from build123d import *

# Parameters (mm, degrees)
SKETCH035_W      = 36
SKETCH035_H      = 4
EXTRUDE033_DEPTH = 2
SKETCH029_W      = 51.25
SKETCH029_H      = 5
EXTRUDE027_DEPTH = 2
SKETCH017_W      = 8.15
SKETCH017_H      = 2.65
EXTRUDE013_DEPTH = 2
SKETCH010_W      = 14.7
SKETCH010_H      = 2.65
SKETCH010_W_2    = 23.15
SKETCH010_H_2    = 3.15
EXTRUDE006_DEPTH = 2
SKETCH_R         = 1.65
EXTRUDE026_DEPTH = 5
SKETCH009_W      = 51.25
SKETCH009_H      = 53
SKETCH009_W_2    = 47.25
SKETCH009_H_2    = 49
EXTRUDE004_DEPTH = 10.25
SKETCH008_W      = 51.25
SKETCH008_H      = 53
EXTRUDE003_DEPTH = 2
SKETCH028_W      = 5
SKETCH028_H      = 5
EXTRUDE025_DEPTH = 5
SKETCH012_R      = 3
EXTRUDE008_DEPTH = 5


with BuildPart() as topcut002:
    # Sketch035 → Extrude033 (new body)
    with BuildSketch(Plane.YZ.offset(49.25)):
        with Locations((26, 7)):
            Rectangle(SKETCH035_W, SKETCH035_H)
    extrude(amount=EXTRUDE033_DEPTH)


with BuildPart() as top006:
    # Sketch029 → Extrude027 (new body)
    with BuildSketch(Plane.XY.offset(12.25)):
        with Locations((25.625, 2.5)):
            Rectangle(SKETCH029_W, SKETCH029_H)
        with Locations((25.625, 50.5)):
            Rectangle(SKETCH029_W, SKETCH029_H)
    extrude(amount=EXTRUDE027_DEPTH)


with BuildPart() as topcut001:
    # Sketch017 → Extrude013 (new body)
    with BuildSketch(Plane.XZ):
        with Locations((37.575, 6.475)):
            Rectangle(SKETCH017_W, SKETCH017_H)
    extrude(amount=-EXTRUDE013_DEPTH)


with BuildPart() as topcuts:
    # Sketch010 → Extrude006 (new body)
    with BuildSketch(Plane.XZ):
        with Locations((10.5, 3.325)):
            Rectangle(SKETCH010_W, SKETCH010_H)
        with Locations((37.575, 3.575)):
            Rectangle(SKETCH010_W_2, SKETCH010_H_2)
    extrude(amount=-EXTRUDE006_DEPTH)


with BuildPart() as topcuts001:
    # Sketch → Extrude026 (new body)
    with BuildSketch(Plane.XY.offset(10.25)):
        with Locations((22.75, 26.5)):
            Circle(SKETCH_R)
    extrude(amount=-EXTRUDE026_DEPTH)

    # Fusion007: union topCut001, topCuts
    add(topcut001.part)
    add(topcuts.part)


with BuildPart() as top:
    # Sketch009 → Extrude004 (new body)
    with BuildSketch(Plane.XY):
        with Locations((25.625, 26.5)):
            Rectangle(SKETCH009_W, SKETCH009_H)
        with Locations((25.625, 26.5)):
            Rectangle(SKETCH009_W_2, SKETCH009_H_2, mode=Mode.SUBTRACT)
    extrude(amount=EXTRUDE004_DEPTH)


with BuildPart() as top_1:
    # Extrude004 placement: moved
    add(top.part.moved(Location((0, 0, 2))))


with BuildPart() as top002:
    # Sketch008 → Extrude003 (new body)
    with BuildSketch(Plane.XY):
        with Locations((25.625, 26.5)):
            Rectangle(SKETCH008_W, SKETCH008_H)
    extrude(amount=EXTRUDE003_DEPTH)


with BuildPart() as top002_1:
    # Extrude003 placement: moved
    add(top002.part.moved(Location((0, 0, 10.25))))

    # Fusion: union top
    add(top_1.part)


with BuildPart() as topaddons:
    # Sketch028 → Extrude025 (new body)
    with BuildSketch(Plane.XY.offset(10.25)):
        with Locations((28.65, 48.5)):
            Rectangle(SKETCH028_W, SKETCH028_H)
        with Locations((46.75, 48.5)):
            Rectangle(SKETCH028_W, SKETCH028_H)
    extrude(amount=-EXTRUDE025_DEPTH)


with BuildPart() as top008:
    # Sketch012 → Extrude008 (new body)
    with BuildSketch(Plane.XY.offset(10.25)):
        with Locations((22.75, 26.5)):
            Circle(SKETCH012_R)
    extrude(amount=-EXTRUDE008_DEPTH)

    # Fusion005: union top002, topAddOns
    add(top002_1.part)
    add(topaddons.part)

    # Cut: cut topCuts001
    add(topcuts001.part, mode=Mode.SUBTRACT)

    # Fusion008: union top006
    add(top006.part)

    # Cut004: cut topCut002
    add(topcut002.part, mode=Mode.SUBTRACT)


solid = top008.part
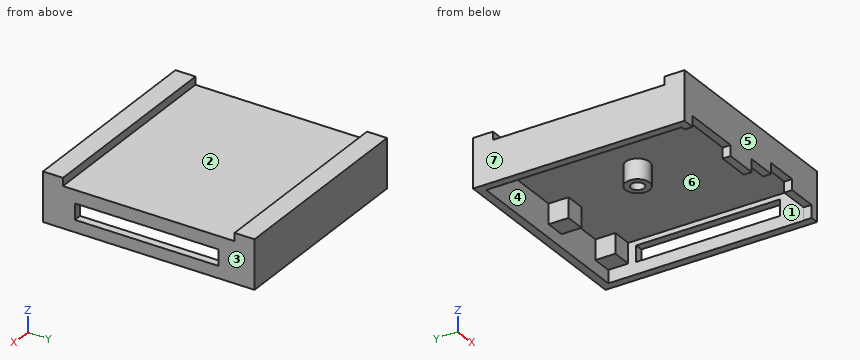
The listing builds one solid part. Answer for the finished solid, in the listing's coordinates (mm). Face numbers are marked on the shaded views. A direction names the side the tool comes from. Coordinates: 2 decimals unless noted, no trailing zeros. Write each loop counter-clockwise with the first axis right and the second up, starting at its lowest first coordinate (ties: lowest second). Pieces come first, ordered by that corner, then holes. Notation, with made-up numbers: (-6.75, 73.5) - (27.25, 73.5) arc R33 cw to (27.25, 106.5) - close; hole circle Ø2 at (25.25, 26). An arc over 180 degrees is marked (long way). Return JSON: item names as keys, results as strings.
1. The part is cut by section B-B on y = 26.5. Determine the outline of the cut face in (x, z), then the cut area to 3 significant figures.
Final values:
{"outline": "(0, 2) - (2, 2) - (2, 10.25) - (19.75, 10.25) - (19.75, 5.25) - (21.1, 5.25) - (21.1, 10.25) - (24.4, 10.25) - (24.4, 5.25) - (25.75, 5.25) - (25.75, 10.25) - (49.25, 10.25) - (49.25, 9) - (51.25, 9) - (51.25, 12.25) - (0, 12.25) - close; (49.25, 2) - (51.25, 2) - (51.25, 5) - (49.25, 5) - close", "area": "141 mm^2"}
2. Consider line 1 along Y through (x, z) = (22.75, 7.9); line 2 along Y through (x, z) = (35, 10); line 3 along X through (y, z) = (14.5, 4.5). Determine where each line is inside the solid, lowest interval first.
Final values:
{"line 1": "0 to 2, 23.5 to 24.85, 28.15 to 29.5, 51 to 53", "line 2": "0 to 2, 51 to 53", "line 3": "0 to 2, 49.25 to 51.25"}
3. The part is cut by section D-D on x = 34.5. Determine the outline of the cut face in (y, z).
Final values:
{"outline": "(0, 7.8) - (2, 7.8) - (2, 10.25) - (51, 10.25) - (51, 2) - (53, 2) - (53, 14.25) - (48, 14.25) - (48, 12.25) - (5, 12.25) - (5, 14.25) - (0, 14.25) - close"}
4. For a pull along X with two mould halves and no side action, classify the marked faces 4, 5, 6 and 7 as +X half, -X half, draft (parallel to the pull), parting line (faces both ways), or undercut.
Final values:
{"face 4": "undercut", "face 5": "draft", "face 6": "undercut", "face 7": "-X half"}
5. The part is cut by section A-A on z = 6.75. Determine the outline of the cut face in (x, y), then the cut area to 3 significant figures.
Final values:
{"outline": "(0, 0) - (33.5, 0) - (33.5, 2) - (2, 2) - (2, 51) - (26.15, 51) - (26.15, 46) - (31.15, 46) - (31.15, 51) - (44.25, 51) - (44.25, 46) - (49.25, 46) - (49.25, 44) - (51.25, 44) - (51.25, 53) - (0, 53) - close; circle Ø6 at (22.75, 26.5); (41.65, 0) - (51.25, 0) - (51.25, 8) - (49.25, 8) - (49.25, 2) - (41.65, 2) - close; hole circle Ø3.3 at (22.75, 26.5)", "area": "382 mm^2"}
6. Which of the six approach directions +Z, -Z, +X, -X, +Y, -Y give full straight-line access (tool end or side, diameter ignored) to the marked faces 1, 2 and 3?
Final values:
{"face 1": "-Z", "face 2": "+Z, +X, -X", "face 3": "+Z, -Z, +X, +Y, -Y"}
7. Each of these flat-tipped pins is pushed along its axis until it touches: pin 1 Ø12 at (x, y) = (36, 34) entering from -Z; pin 2 Ø0.6 at (x, y) = (46, 0.5) entering from -Z; pin 3 Ø21.5 at (x, y) = (36.5, 30) entering from +Z. Where does it stop, or does it pass through?
Final values:
{"pin 1": "z = 10.25", "pin 2": "z = 5.15", "pin 3": "z = 12.25"}
8. The part is cut by section C-C on z = 3.75. Determine the outline of the cut face in (x, y).
Final values:
{"outline": "(0, 0) - (3.15, 0) - (3.15, 2) - (2, 2) - (2, 51) - (49.25, 51) - (49.25, 2) - (49.15, 2) - (49.15, 0) - (51.25, 0) - (51.25, 53) - (0, 53) - close; (17.85, 0) - (26, 0) - (26, 2) - (17.85, 2) - close"}
